Verification items for the finished model (mm, model axes). A direction names the side the tool comes from. Coordinates: 2 decimals unless noted, no trailing zeros. Order: outer loops, then holes, each group sorted by start corner. A loop starts at its lowest first (then second) coordinate and runs counter-clockwise, first axis right, second up. Notation, with made-up numbers: (-3, 30) -> (3, 30) arc R20 ccw to (3, 36) -> close; hole circle Ø5 at (22.5, 84). An arc over 180 degrees is marked (long way). Write item = value, one per line. Start each with the question number.
1. Set-up check for faces 1 (the flat face through (8, -13, 30.48)), 2 (the flat face through (-4.33, -13, -48)), 3 (the flat face through (-22, -13, -30.48)): record each of +Z, -Z, +X, -X, +Y, -Y from which the full face is reachable in a straight line by a thin tool's end or side.
2. Cross-section at B-B on z = 36. Record the cut outline in (x, y).
3. Cross-section at A-A on z = -15. Record the cut outline in (x, y), plus the area to 3 significant figures.
4. Release check for a two-part mould opening along X. For faces 4 (the flat face through (-12, -13, 40.64)), 5 (the flat face through (-88.15, -13, -40)), 6 (the flat face through (-12, -13, 0)) record: +X half, -X half, draft (parallel to the pull), parting line (faces both ways), or undercut.
5. Go/stop test with flat-tipped pins: P1, Ø11, axis at x = -70.5, y = -13, coming from the -Z side; P2, Ø8, axis at x = -55.5, y = -9, coming from the -Z side; P3, Ø12, axis at y = -10, z = -4.5, coming from the +X side. Record where each tip stops, or that it passes through.
6. Thickness scan on line 1 along X through (y, z) = (-0.75, 28); line 2 along Z through (x, y) = (-66, -13); line 3 along X through (y, z) = (-19.25, 49). Record the ranges inside material, lowest first. Write a range as from..to.
from build123d import *

# Parameters (mm, degrees)
F1_DEPTH = 25.4
F2_T     = -2.54


with BuildPart() as f1:
    # F0 (on Front) → F1 (new body)
    with BuildSketch(Plane.XZ):
        Polygon((-6.8695716643, -40.64), (-6.8695716643, -60.96), (23.6104283357, -60.96), (23.6104283357, -30.48), (3.2904283357, -30.48), (3.2904283357, -20.32), (-6.8695716643, -20.32), (-17.0295716643, -20.32), (-27.1895716643, -20.32), (-27.1895716643, -30.48), (-17.0295716643, -30.48), (-17.0295716643, -40.64), align=None)
        Polygon((-17.0295716643, -20.32), (-6.8695716643, -20.32), (-6.8695716643, -10.16), (-17.0295716643, -10.16), (-17.0295716643, 0), (-6.8695716643, 0), (-6.8695716643, 10.16), (3.2904283357, 10.16), (3.2904283357, 30.48), (13.4504283357, 30.48), (13.4504283357, 50.8), (-6.8695716643, 50.8), (-6.8695716643, 40.64), (-17.0295716643, 40.64), (-17.0295716643, 30.48), (-27.1895716643, 30.48), (-27.1895716643, 20.32), (-37.3495716643, 20.32), (-47.5095716643, 20.32), (-57.6695716643, 20.32), (-77.9895716643, 20.32), (-77.9895716643, 10.16), (-67.8295716643, 10.16), (-67.8295716643, 0), (-57.6695716643, 0), (-57.6695716643, -10.16), (-57.6695716643, -20.32), (-37.3495716643, -20.32), (-27.1895716643, -20.32), align=None)
        Polygon((-37.3495716643, -30.48), (-37.3495716643, -20.32), (-57.6695716643, -20.32), (-57.6695716643, -10.16), (-67.8295716643, -10.16), (-67.8295716643, -20.32), (-77.9895716643, -20.32), (-77.9895716643, -30.48), (-88.1495716643, -30.48), (-88.1495716643, -50.8), (-67.8295716643, -50.8), (-67.8295716643, -40.64), (-47.5095716643, -40.64), (-47.5095716643, -30.48), align=None)
        Polygon((-88.1495716643, 20.32), (-77.9895716643, 20.32), (-57.6695716643, 20.32), (-47.5095716643, 20.32), (-37.3495716643, 20.32), (-37.3495716643, 30.48), (-47.5095716643, 30.48), (-67.8295716643, 30.48), (-88.1495716643, 30.48), align=None)
        Polygon((-98.3095716643, 30.48), (-88.1495716643, 30.48), (-67.8295716643, 30.48), (-47.5095716643, 30.48), (-47.5095716643, 40.64), (-57.6695716643, 40.64), (-77.9895716643, 40.64), (-98.3095716643, 40.64), align=None)
        Polygon((-108.4695716643, 40.64), (-98.3095716643, 40.64), (-77.9895716643, 40.64), (-57.6695716643, 40.64), (-57.6695716643, 50.8), (-67.8295716643, 50.8), (-88.1495716643, 50.8), (-108.4695716643, 50.8), align=None)
        Polygon((-118.6295716643, 50.8), (-108.4695716643, 50.8), (-88.1495716643, 50.8), (-67.8295716643, 50.8), (-67.8295716643, 60.96), (-77.9895716643, 60.96), (-98.3095716643, 60.96), (-118.6295716643, 60.96), align=None)
        Polygon((-128.7895716643, 60.96), (-118.6295716643, 60.96), (-98.3095716643, 60.96), (-77.9895716643, 60.96), (-77.9895716643, 71.12), (-88.1495716643, 71.12), (-88.1495716643, 81.28), (-98.3095716643, 81.28), (-98.3095716643, 91.44), (-108.4695716643, 91.44), (-108.4695716643, 101.6), (-138.9495716643, 101.6), (-138.9495716643, 71.12), (-128.7895716643, 71.12), align=None)
    extrude(amount=F1_DEPTH)

    # F2
    f2_openings = [f1.faces().sort_by_distance(p)[0] for p in [
        (-54.908702, -25.4, 17.55913),
        (-54.908702, 0, 17.55913),
    ]]
    offset(amount=F2_T, openings=f2_openings, kind=Kind.INTERSECTION)


solid = f1.part
Worked out:
q1.face_1 = +X, +Y, -Y
q1.face_2 = +Y, -Y
q1.face_3 = -Z, +Y, -Y
q2.outline = (-98.31, -25.4) -> (-95.77, -25.4) -> (-95.77, 0) -> (-98.31, 0) -> close; (-50.05, -25.4) -> (-47.51, -25.4) -> (-47.51, 0) -> (-50.05, 0) -> close; (-17.03, -25.4) -> (-14.49, -25.4) -> (-14.49, 0) -> (-17.03, 0) -> close; (10.91, -25.4) -> (13.45, -25.4) -> (13.45, 0) -> (10.91, 0) -> close
q3.outline = (-67.83, -25.4) -> (-65.29, -25.4) -> (-65.29, 0) -> (-67.83, 0) -> close; (-9.41, -25.4) -> (-6.87, -25.4) -> (-6.87, 0) -> (-9.41, 0) -> close
q3.area = 129 mm²
q4.face_4 = undercut
q4.face_5 = -X half
q4.face_6 = draft
q5.P1 = -50.8
q5.P2 = -40.64
q5.P3 = -6.87
q6.line_1 = -88.15..-85.61, -50.05..-37.35, -27.19..-14.49, 0.75..3.29
q6.line_2 = -40.64..-38.1, -22.86..-10.16, 0..12.7, 48.26..50.8
q6.line_3 = -108.47..-105.93, -70.37..-57.67, -6.87..13.45
